Autodesk Inventor part; units mm, degrees
ref_plane "Start Plane" through (0, 0, 0) normal (0, 0, 1) x (1, 0, 0)
ref_plane "End Plane" through (0, 0, 690) normal (0, 0, 1) x (1, 0, 0)
ref_plane "YZ Plane" through (0, 0, 0) normal (1, 0, 0) x (0, 1, 0)
ref_plane "Start Plane" through (0, 0, 0) normal (0, 0, 1) x (1, 0, 0)
ref_plane "End Plane" through (0, 0, 690) normal (0, 0, 1) x (1, 0, 0)
sketch "Sketch" plane through (0, 0, 0) normal (0, 0, 1) x (1, 0, 0)
  line L0 (25.4, 0) -> (0, 0)
  line L1 (0, 0) -> (0, 25.4)
  line L2 (0, 25.4) -> (1.651, 25.4)
  line L3 (3.175, 23.876) -> (3.175, 6.477)
  line L4 (6.477, 3.175) -> (23.876, 3.175)
  line L5 (25.4, 1.651) -> (25.4, 0)
  line L6 (0, -11.0414) -> (0, 31.5385) construction
  line L7 (-11.0414, 0) -> (31.5385, 0) construction
  arc A0 (3.175, 6.477) -> (6.477, 3.175) centre (6.477, 6.477) ccw
  arc A1 (3.175, 23.876) -> (1.651, 25.4) centre (1.651, 23.876) ccw
  arc A2 (25.4, 1.651) -> (23.876, 3.175) centre (23.876, 1.651) ccw
  line L8 (0, 40.0545) -> (0, -19.5574) construction
  line L9 (-19.5574, 0) -> (40.0545, 0) construction
  point P0 (3.175, 25.4)
  point P1 (3.175, 3.175)
  point P2 (25.4, 3.175)
  dimension "d0" = 25.4
  dimension "d1" = 25.4
  dimension "d2" = 3.175
  dimension "d3" = 3.175
  dimension "d10" = 0
  dimension "d11" = 0
  dimension "d14" = 3.302
  dimension "d15" = 1.524
extrude "Body" add sketch "Sketch" along normal up to surface (690 mm away) from surface at 0
sketch "Sketch3" plane through (0, 0, 0) normal (0, 0, 1) x (1, 0, 0)
  line L0 (0, 0) -> (10, 0)
ref_plane "Work Plane3" through (0, 0, 0) normal (0, -1, 0) x (1, 0, 0)
sketch "Sketch4" plane through (0, 0, 0) normal (0, -1, 0) x (1, 0, 0)
  line L0 (-2, 0) -> (12, 0)
  line L1 (-2, 690) -> (12, 690)
  dimension "d17" = 690
equation "\"d0\" = G_H"
equation "\"d1\" = G_H"
equation "\"d2\" = G_T"
equation "\"d3\" = G_T"
equation "\"d14\" = G_IR"
equation "\"d15\" = G_ER"
equation "\"d4\" = G_L"
equation "\"G_H\" = 25.4"
equation "\"G_T\" = 3.175"
equation "\"G_ER\" = 1.524"
equation "\"G_IR\" = 3.302"
equation "\"G_L\" = d17"
equation "\"ex\" = 0"
equation "\"G_OFFSET_START\" = 0"
equation "\"G_OFFSET_END\" = 0"
equation "\"d13\" = G_OFFSET_END + B_L"
equation "\"B_L\" = 690"
properties part number "AISC - L 1 x 1 x 1/8 - 27.165" material "Steel, Mild"
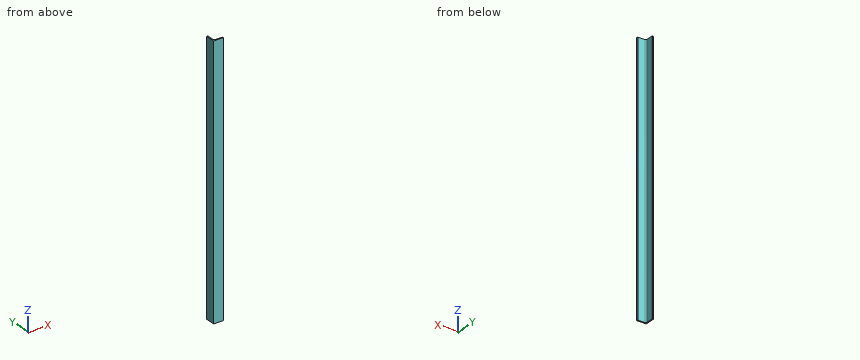
The listing builds one solid part. Answer for the finished solid, in the listing's coordinates (mm). Give positions to 0.01 mm unless a question says otherwise; leave off trailing zeros. Loops run counter-clockwise (first coordinate to the right, second up) from the corner with the lowest first, then second, coordinate; pieces in that order, holes last. Notation, with made-up numbers: M -28.5,8 L -24.5,8 A8 ccw -24.5,20 Z; hole C 15,36 d3. An arc over 180 degrees is marked long. One line per item, written item: value.
Q1. A cutting plane is placed at A-A on z = 192. Determine the outline of the cut face in (x, y) (3 decimals).
Working result:
outline: M 0,0 L 25.4,0 L 25.4,1.651 A1.524 ccw 23.876,3.175 L 6.477,3.175 A3.302 cw 3.175,6.477 L 3.175,23.876 A1.524 ccw 1.651,25.4 L 0,25.4 Z
Q2. Flat-ended cylindrical pins translate along their axes: P1, Ø14, axis at x = 15, z = 226.5, coming from the +Y side (3 decimals); P2, Ø12, axis at y = 20, z = 425.5, coming from the +X side (3 decimals). Find the tip coordinate at first contact, or state that the pin passes through.
Working result:
P1: stops at y = 3.175
P2: stops at x = 3.175
Q3. Find the intervals of material crossed by line 1 (X direction, y = 10, z = 110) (3 decimals); line 2 (X direction, y = 1.75, z = 462), in increasing order. Write a range as from..to.
Working result:
line 1: x = 0..3.175
line 2: x = 0..25.4
Q4. A cutting plane is placed at B-B on x = 17.5. Determine the outline of the cut face in (y, z) (3 decimals).
Working result:
outline: M 0,0 L 3.175,0 L 3.175,690 L 0,690 Z
